Here's how the part is built. I have some questions about the finished solid (model axes, mm). A direction names the side the tool comes from. Coordinates: 2 decimals unless noted, no trailing zeros. Loops run counter-clockwise (first coordinate to the right, second up) from the corner with the lowest first, then second, coordinate; pieces in that order, holes last. Notation, with made-up numbers: (-3.5, 47.5) - (11.5, 47.5) arc R19 cw to (11.5, 73.5) - close; hole circle Ø4 at (79, 63.5). An arc over 180 degrees is marked (long way). Use a Markdown table: item, result.
```python
from build123d import *

# Parameters (mm, degrees)
SKETCH1_W                = 130
SKETCH1_H                = 80
BOSS_EXTRUDE1_DEPTH      = 3
BOSS_EXTRUDE2_DEPTH      = 5
BOSS_EXTRUDE2_DEPTH_BACK = 5
SKETCH3_W                = 4
SKETCH3_H                = 10
BOSS_EXTRUDE3_DEPTH      = 2
SKETCH4_W                = 10
SKETCH4_H                = 2
BOSS_EXTRUDE4_DEPTH      = 5


with BuildPart() as part:
    # Sketch1 → Boss-Extrude1 (new body)
    with BuildSketch(Plane(origin=(0, 0, 0), x_dir=(1, 0, 0), z_dir=(0, 1, 0))):
        Rectangle(SKETCH1_W, SKETCH1_H)
    extrude(amount=BOSS_EXTRUDE1_DEPTH)

    # Sketch2 → Boss-Extrude2 (add, two sides: drawn at the far end of the back side and taken through both)
    with BuildSketch(Plane.XY.offset(-BOSS_EXTRUDE2_DEPTH_BACK)):
        with BuildLine():
            Line((63.5, 1.5), (63.5, -6.205455333))
            ThreePointArc((63.5, -6.205455333), (63.792893219, -6.912562114), (64.5, -7.205455333))
            Line((64.5, -7.205455333), (67.5, -7.205455333))
            ThreePointArc((67.5, -7.205455333), (68.207106781, -6.912562114), (68.5, -6.205455333))
            Line((68.5, -6.205455333), (68.5, 1.5))
            Line((68.5, 1.5), (72.74730308, 1.5))
            Line((72.74730308, 1.5), (72.74730308, 3))
            Line((72.74730308, 3), (67, 3))
            Line((67, 3), (67, -5.105455333))
            ThreePointArc((67, -5.105455333), (66.824264069, -5.529719402), (66.4, -5.705455333))
            Line((66.4, -5.705455333), (65.6, -5.705455333))
            ThreePointArc((65.6, -5.705455333), (65.175735931, -5.529719402), (65, -5.105455333))
            Line((65, -5.105455333), (65, 1.5))
            Line((65, 1.5), (63.5, 1.5))
        make_face()
    extrude(amount=BOSS_EXTRUDE2_DEPTH + BOSS_EXTRUDE2_DEPTH_BACK)

    # Sketch3 → Boss-Extrude3 (add)
    with BuildSketch(Plane.XZ):
        with Locations((-63, 24.089900089)):
            Rectangle(SKETCH3_W, SKETCH3_H)
        with Locations((-63, -24.089900089)):
            Rectangle(SKETCH3_W, SKETCH3_H)
    extrude(amount=BOSS_EXTRUDE3_DEPTH)

    # Sketch4 → Boss-Extrude4 (add)
    with BuildSketch(Plane.ZY.offset(65)):
        with Locations((-24.089900089, -1)):
            Rectangle(SKETCH4_W, SKETCH4_H)
        with Locations((24.089900089, -1)):
            Rectangle(SKETCH4_W, SKETCH4_H)
    extrude(amount=BOSS_EXTRUDE4_DEPTH)


solid = part.part
```
Q1. I want a section at C-C, the plane z = 15.5. Write out the boundary of the cut face in (x, y), then the cut area to 3 significant figures.
Check values:
| item | result |
|---|---|
| outline | (-65, 0) - (65, 0) - (65, 3) - (-65, 3) - close |
| area | 390 mm^2 |
Q2. If we mould it in two halves opening along X, with no side actions, what happens to faces 5 (the face through (67, -1, 0)), 6 (the face through (68.5, -2, 0)), 7 (the face through (-67, 0, -24))? For each: pulls with the +X half, pulls with the -X half, needs draft (parallel to the pull), parting line crosses it, or undercut.
Check values:
| item | result |
|---|---|
| face 5 | undercut |
| face 6 | pulls with the +X half |
| face 7 | needs draft |
Q3. Which directions (+Z, -Z, +X, -X, +Y, -Y) give clear straight access to the entire face, cutting with the end or side of a thin tool? Please do faces 1 (the face through (65, 1, 1)), 2 (the face through (71, 1.5, 0)), 3 (the face through (-67, 0, 24)), 4 (the face through (63.5, -3, 0)).
Check values:
| item | result |
|---|---|
| face 1 | +Z, -Z, +Y |
| face 2 | +Z, -Z, +X, -Y |
| face 3 | +Z, -Z, -X, +Y |
| face 4 | +Z, -Z, -X, -Y |
Q4. Will these pins go through, and if not, where does the flat tip stop? P1, Ø4, axis at y = -3, z = -2, coming from the -X side; P2, Ø4, axis at y = 1.5, z = -1.5, coming from the -X side; P3, Ø0.6, axis at x = -67.5, y = -1, coming from the +Z side; P4, Ø2, axis at y = -3, z = 17.5, coming from the -X side.
Check values:
| item | result |
|---|---|
| P1 | x = 63.5 |
| P2 | x = -65 |
| P3 | z = 29.09 |
| P4 | through |
Q5. Please list where these lines run through material, in increasing order: L1, parallel to X at y = 2.25, z = 1; L2, parallel to Y at x = -60.5, z = 35; L3, parallel to X at y = -2.5, z = -1.5. Write a range as from..to.
Check values:
| item | result |
|---|---|
| L1 | -65..65, 67..72.75 |
| L2 | 0..3 |
| L3 | 63.5..65, 67..68.5 |
Q6. I want a section at B-B, the plane x = -38.5. Write out the boundary of the cut face in (y, z), then the cut area to 3 significant figures.
Check values:
| item | result |
|---|---|
| outline | (0, -40) - (3, -40) - (3, 40) - (0, 40) - close |
| area | 240 mm^2 |
Q7. I want a section at A-A, the plane z = -23.5. Write out the boundary of the cut face in (x, y).
Check values:
| item | result |
|---|---|
| outline | (-70, -2) - (-61, -2) - (-61, 0) - (65, 0) - (65, 3) - (-65, 3) - (-65, 0) - (-70, 0) - close |
